```python
from build123d import *

# Parameters (mm, degrees)
Y_KSEKLIK_EKSTR_ZYON1_DEPTH = 9
Y_KSEKLIK_EKSTR_ZYON2_DEPTH = 6
IZIM4_R                     = 1.5
IZIM4_R_2                   = 2.5
KES_EKSTR_ZYON2_DEPTH       = 6.5
IZIM5_W                     = 14
IZIM5_H                     = 15
Y_KSEKLIK_EKSTR_ZYON3_DEPTH = 5
Y_KSEKLIK_EKSTR_ZYON4_DEPTH = 7
IZIM3_W                     = 7.2
IZIM3_H                     = 2
IZIM3_W_2                   = 2
IZIM3_H_2                   = 8.3
KES_EKSTR_ZYON3_DEPTH       = 3
IZIM8_R                     = 1.5
KES_EKSTR_ZYON5_DEPTH       = 10
IZIM9_R                     = 2.5
IZIM9_R_2                   = 4
KES_EKSTR_ZYON6_DEPTH       = 2
IZIM11_R                    = 2.5
KES_EKSTR_ZYON8_DEPTH       = 2
KES_EKSTR_ZYON9_START       = -10
KES_EKSTR_ZYON9_DEPTH       = 10
IZIM14_W                    = 14
IZIM14_H                    = 3
Y_KSEKLIK_EKSTR_ZYON5_DEPTH = 5


with BuildPart() as part:
    # izim1 → Y_kseklik-Ekstr_zyon1 (new body)
    with BuildSketch(Plane.XY):
        with BuildLine():
            Line((17, 7), (17, -7))
            ThreePointArc((17, -7), (14.071067812, -14.071067812), (7, -17))
            Line((7, -17), (-7, -17))
            ThreePointArc((-7, -17), (-14.071067812, -14.071067812), (-17, -7))
            Line((-17, -7), (-17, 7))
            ThreePointArc((-17, 7), (-14.071067812, 14.071067812), (-7, 17))
            Line((-7, 17), (7, 17))
            ThreePointArc((7, 17), (14.071067812, 14.071067812), (17, 7))
        make_face()
        with BuildLine():
            Line((-7, 12), (7, 12))
            ThreePointArc((7, 12), (10.535533906, 10.535533906), (12, 7))
            Line((12, 7), (12, -7))
            ThreePointArc((12, -7), (10.535533906, -10.535533906), (7, -12))
            Line((7, -12), (-7, -12))
            ThreePointArc((-7, -12), (-10.535533906, -10.535533906), (-12, -7))
            Line((-12, -7), (-12, 7))
            ThreePointArc((-12, 7), (-10.535533906, 10.535533906), (-7, 12))
        make_face(mode=Mode.SUBTRACT)
    extrude(amount=Y_KSEKLIK_EKSTR_ZYON1_DEPTH)

    # izim2 → Y_kseklik-Ekstr_zyon2 (add)
    with BuildSketch(Plane.XY):
        with BuildLine():
            Line((-7, -12), (7, -12))
            ThreePointArc((7, -12), (10.535533906, -10.535533906), (12, -7))
            Line((12, -7), (12, 7))
            ThreePointArc((12, 7), (10.535533906, 10.535533906), (7, 12))
            Line((7, 12), (-7, 12))
            ThreePointArc((-7, 12), (-10.535533906, 10.535533906), (-12, 7))
            Line((-12, 7), (-12, -7))
            ThreePointArc((-12, -7), (-10.535533906, -10.535533906), (-7, -12))
        make_face()
    extrude(amount=Y_KSEKLIK_EKSTR_ZYON2_DEPTH)

    # izim4 → Kes-Ekstr_zyon2 (cut)
    with BuildSketch(Plane.XY.offset(6)):
        with Locations((0, 9)):
            Circle(IZIM4_R)
        Circle(IZIM4_R_2)
        with Locations((9, 0)):
            Circle(IZIM4_R)
        with Locations((0, -9)):
            Circle(IZIM4_R)
        with Locations((-9, 0)):
            Circle(IZIM4_R)
    extrude(amount=-KES_EKSTR_ZYON2_DEPTH, mode=Mode.SUBTRACT)

    # izim5 → Y_kseklik-Ekstr_zyon3 (add)
    with BuildSketch(Plane.XY):
        with Locations((0, -24.5)):
            Rectangle(IZIM5_W, IZIM5_H)
    extrude(amount=Y_KSEKLIK_EKSTR_ZYON3_DEPTH)

    # izim6 → Y_kseklik-Ekstr_zyon4 (add, symmetric)
    with BuildSketch(Plane(origin=(0, 0, 0), x_dir=(0, 0, -1), z_dir=(1, 0, 0))):
        with BuildLine():
            Line((0, -32), (-5, -32))
            Line((-5, -32), (-5, -42))
            ThreePointArc((-5, -42), (5, -52), (15, -42))
            Line((15, -42), (15, -32))
            Line((15, -32), (10, -32))
            Line((10, -32), (10, -42))
            ThreePointArc((10, -42), (5, -47), (0, -42))
            Line((0, -42), (0, -32))
        make_face()
    extrude(amount=Y_KSEKLIK_EKSTR_ZYON4_DEPTH, both=True)

    # izim3 → Kes-Ekstr_zyon3 (cut)
    with BuildSketch(Plane.XY.offset(6)):
        with Locations((8.4, 2.7)):
            Rectangle(IZIM3_W, IZIM3_H)
        with Locations((2.7, 7.85)):
            Rectangle(IZIM3_W_2, IZIM3_H_2)
        with Locations((-2.7, 7.85)):
            Rectangle(IZIM3_W_2, IZIM3_H_2)
        with Locations((-8.4, 2.7)):
            Rectangle(IZIM3_W, IZIM3_H)
        with Locations((-8.4, -2.7)):
            Rectangle(IZIM3_W, IZIM3_H)
        with Locations((-2.7, -7.85)):
            Rectangle(IZIM3_W_2, IZIM3_H_2)
        with Locations((2.7, -7.85)):
            Rectangle(IZIM3_W_2, IZIM3_H_2)
        with Locations((8.4, -2.7)):
            Rectangle(IZIM3_W, IZIM3_H)
    extrude(amount=-KES_EKSTR_ZYON3_DEPTH, mode=Mode.SUBTRACT)

    # izim8 → Kes-Ekstr_zyon5 (cut)
    with BuildSketch(Plane.XY.offset(-10)):
        with Locations((-4, -37)):
            Circle(IZIM8_R)
        with Locations((4, -37)):
            Circle(IZIM8_R)
    extrude(amount=-KES_EKSTR_ZYON5_DEPTH, mode=Mode.SUBTRACT)

    # izim9 → Kes-Ekstr_zyon6 (cut)
    with BuildSketch(Plane(origin=(0, 0, 0), x_dir=(-1, 0, 0), z_dir=(0, 0, -1))):
        with Locations((0, 9)):
            Circle(IZIM9_R)
        Circle(IZIM9_R_2)
        with Locations((9, 0)):
            Circle(IZIM9_R)
        with Locations((0, -9)):
            Circle(IZIM9_R)
        with Locations((-9, 0)):
            Circle(IZIM9_R)
    extrude(amount=-KES_EKSTR_ZYON6_DEPTH, mode=Mode.SUBTRACT)

    # izim11 → Kes-Ekstr_zyon8 (cut)
    with BuildSketch(Plane(origin=(0, 0, -15), x_dir=(-1, 0, 0), z_dir=(0, 0, -1))):
        with Locations((-4, -37)):
            Circle(IZIM11_R)
        with Locations((4, -37)):
            Circle(IZIM11_R)
    extrude(amount=-KES_EKSTR_ZYON8_DEPTH, mode=Mode.SUBTRACT)

    # izim12 → Kes-Ekstr_zyon9 (cut)
    with BuildSketch(Plane.XY.offset(9).offset(KES_EKSTR_ZYON9_START)):
        with BuildLine():
            Line((7, 17), (-7, 17))
            ThreePointArc((-7, 17), (-14.071067812, 14.071067812), (-17, 7))
            Line((-17, 7), (-17, -7))
            ThreePointArc((-17, -7), (-14.071067812, -14.071067812), (-7, -17))
            Line((-7, -17), (7, -17))
            ThreePointArc((7, -17), (14.071067812, -14.071067812), (17, -7))
            Line((17, -7), (17, 7))
            ThreePointArc((17, 7), (14.071067812, 14.071067812), (7, 17))
        make_face()
        with BuildLine():
            Line((7, 14), (-7, 14))
            ThreePointArc((-7, 14), (-11.949747468, 11.949747468), (-14, 7))
            Line((-14, 7), (-14, -7))
            ThreePointArc((-14, -7), (-11.949747468, -11.949747468), (-7, -14))
            Line((-7, -14), (7, -14))
            ThreePointArc((7, -14), (11.949747468, -11.949747468), (14, -7))
            Line((14, -7), (14, 7))
            ThreePointArc((14, 7), (11.949747468, 11.949747468), (7, 14))
        make_face(mode=Mode.SUBTRACT)
    extrude(amount=KES_EKSTR_ZYON9_DEPTH, mode=Mode.SUBTRACT)


with BuildPart() as kes_ekstr_zyon9_piece_1:
    # of the separate pieces the step leaves, piece 1, a body of its own (kes_ekstr_zyon9_pieces)
    add(part.part.solids().sort_by_distance((7, 14, 0))[0])



with BuildPart() as kes_ekstr_zyon9_piece_2:
    # of the separate pieces the step leaves, piece 2, a body of its own (kes_ekstr_zyon9_pieces)
    add(part.part.solids().sort_by_distance((-7, -42, 0))[0])


with BuildPart() as kes_ekstr_zyon9_piece_1_1:
    add(kes_ekstr_zyon9_piece_1.part)

    add(kes_ekstr_zyon9_piece_2.part)  # Y_kseklik-Ekstr_zyon5 merges Kes-Ekstr_zyon9 piece 2
    # izim14 → Y_kseklik-Ekstr_zyon5 (add)
    with BuildSketch(Plane.XY):
        with Locations((0, -15.5)):
            Rectangle(IZIM14_W, IZIM14_H)
    extrude(amount=Y_KSEKLIK_EKSTR_ZYON5_DEPTH)


solid = kes_ekstr_zyon9_piece_1_1.part
```
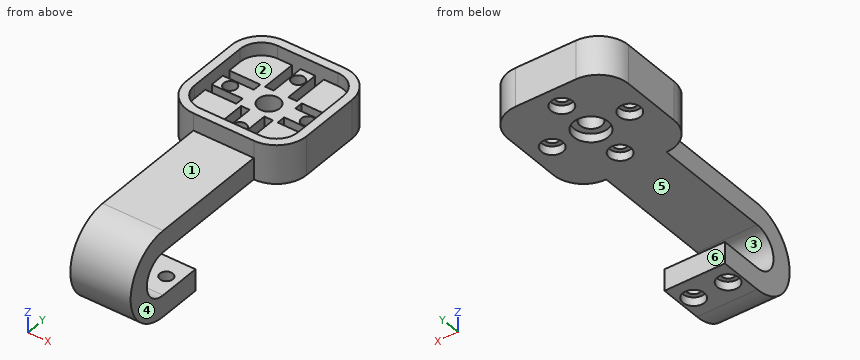
CAD build for the part. Positions are in the model's coordinates, mm. Face numbers are marked on the shaded views. A direction names the side the tool comes from. Round coordinates to 2 decimals unless told otherwise and drop trailing zeros. Write each loop counter-clockwise with the first axis right and the second up, starting at its lowest first coordinate (ties: lowest second). Pieces come first, ordered by that corner, then holes. Notation, with made-up numbers: (32.5, -7) - (49.5, -7) arc R12 cw to (49.5, 13) - close; hole circle Ø4 at (65, 24.5). An arc over 180 degrees is marked (long way). Write item = value, one per line. Start each with the question number.
Q1. Band-saw the part on B-B (x = 9.25). Give the cut face in (y, z), then the cut area to 3 significant figures.
Q2. Band-saw the part on A-A (y = -37). Give the cut face in (x, z).
Q3. Probe L1, parallel to Z at x = 4.75, y = -41; L2, parallel to Y at x = 0, z = 0.9; L3, parallel to Z at x = -12.25, y = -5.5. List the from-to ranges inside material, lowest first. Write a range as from..to.
Q4. Band-saw the part on C-C (z = 6.75). Give the cut face in (x, y), then the cut area to 3 significant figures.
Q5. Drop flat-ended pins along their axis: pin 1 (1 mm diameter, centred on x = 3, y = 7.5, fed in from +Z); pin 2 (5 mm diameter, centred on x = -3, y = -10, fed in from -Z); pin 3 (2.5 mm diameter, centred on y = 8.5, z = 5, fed in from -X). Give the stop position or say it passes through.
Q6. Band-saw the part on D-D (y = -9). Give the cut face in (x, z).
Q7. Which spindle directions (+Z, -Z, +X, -X, +Y, -Y) get a long thin tool onto all of the face, cutting with end or side? Do the marked faces 4, 5 and 6. Say none if no direction does.
Q8. Mould opens along Y. For the marked faces 1, 2 and 3 say: pulls with the +Y half, pulls with the -Y half, needs draft (parallel to the pull), parting line crosses it, or undercut.
Answers below:
q1.outline = (-13.63, 0) - (-2.49, 0) - (-2.49, 2) - (-1.48, 2) - (-1.48, 6) - (-1.7, 6) - (-1.7, 3) - (-3.7, 3) - (-3.7, 6) - (-11.47, 6) - (-11.47, 9) - (-13.63, 9) - close; (1.48, 2) - (2.49, 2) - (2.49, 0) - (13.63, 0) - (13.63, 9) - (11.47, 9) - (11.47, 6) - (3.7, 6) - (3.7, 3) - (1.7, 3) - (1.7, 6) - (1.48, 6) - close
q1.area = 143 mm2
q2.outline = (-7, -15) - (-6.5, -15) - (-6.5, -13) - (-5.5, -13) - (-5.5, -10) - (-7, -10) - close; (-7, 0) - (7, 0) - (7, 5) - (-7, 5) - close; (-2.5, -13) - (-1.5, -13) - (-1.5, -15) - (1.5, -15) - (1.5, -13) - (2.5, -13) - (2.5, -10) - (-2.5, -10) - close; (5.5, -13) - (6.5, -13) - (6.5, -15) - (7, -15) - (7, -10) - (5.5, -10) - close
q3.L1 = -15..-10, 0..5
q3.L2 = -50.07..-11.5, -6.5..-4, 4..6.5, 11.5..14
q3.L3 = 0..9
q4.outline = (-14, -7) arc R7 ccw to (-7, -14) - (7, -14) arc R7 ccw to (14, -7) - (14, 7) arc R7 ccw to (7, 14) - (-7, 14) arc R7 ccw to (-14, 7) - close; hole (-12, -7) arc R5 ccw to (-7, -12) - (7, -12) arc R5 ccw to (12, -7) - (12, 7) arc R5 ccw to (7, 12) - (-7, 12) arc R5 ccw to (-12, 7) - close
q4.area = 187 mm2
q5.pin_1 = 3
q5.pin_2 = 0
q5.pin_3 = -14
q6.outline = (-13.71, 0) - (-2.5, 0) - (-2.5, 2) - (-1.5, 2) - (-1.5, 6) - (-1.7, 6) - (-1.7, 3) - (-3.7, 3) - (-3.7, 6) - (-11.58, 6) - (-11.58, 9) - (-13.71, 9) - close; (1.5, 2) - (2.5, 2) - (2.5, 0) - (13.71, 0) - (13.71, 9) - (11.58, 9) - (11.58, 6) - (3.7, 6) - (3.7, 3) - (1.7, 3) - (1.7, 6) - (1.5, 6) - close
q7.face_4 = +Z, -Z, +X, -Y
q7.face_5 = +X, -X, +Y
q7.face_6 = -Z, +X, -X, +Y
q8.face_1 = needs draft
q8.face_2 = undercut
q8.face_3 = pulls with the +Y half
